Check sheet for the modelled part. Datum: model origin and axes. Units: mm. Face numbers are marked on the shaded views. A direction names the side the tool comes from. Round coordinates to 2 decimals unless told otherwise and drop trailing zeros. One line per question, with ' | ' between items.
Autodesk Inventor part; units mm, degrees
ref_plane "YZ Plane" through (0, 0, 0) normal (1, 0, 0) x (0, 1, 0)
ref_plane "XZ Plane" through (0, 0, 0) normal (0, 1, 0) x (-1, 0, 0)
ref_plane "XY Plane" through (0, 0, 0) normal (0, 0, 1) x (1, 0, 0)
sketch "Skizze1" plane through (0, 0, 0) normal (0, 0, 1) x (1, 0, 0)
  line L0 (-91, 0) -> (91, 0) construction
  circle A0 centre (0, 0) radius 65
  line L1 (-9.5, 25) -> (9.5, 25)
  line L2 (9.5, 25) -> (9.5, 22)
  line L3 (9.5, 22) -> (-9.5, 22)
  line L4 (-9.5, 22) -> (-9.5, 25)
  line L5 (1.5, 22) -> (-1.5, 22)
  line L6 (-1.5, 22) -> (-1.5, 15)
  line L7 (-1.5, 15) -> (1.5, 15)
  line L8 (1.5, 15) -> (1.5, 22)
  circle A1 centre (0, 0) radius 10
  line L9 (0, 91) -> (0, -91) construction
  dimension "d9" = 130
  dimension "d10" = 3
  dimension "d14" = 19
  dimension "d23" = 7
  dimension "d62" = 20
  dimension "d149" = 25
extrude "Extrusion3" add sketch "Skizze1" against normal blind 7 contours L1 L2 L3 L4 | L3 L8 L7 L6
chamfer "Fase2" distance 3 distance2 7 1 edges at (-9.5, 23.5, -7) measured on face at (-0.5, 24, -7)
chamfer "Fase3" distance 3 distance2 7 1 edges at (9.5, 23.5, -7) measured on face at (1.5, 24, -7)
fillet "Rundung1" radius 4 2 edges at (-6.5001, 23.5, -7) (6.5001, 23.5, -7)
sketch "Skizze2" plane through (-9.5, 25, 0) normal (0, 1, 0) x (1, 0, 0)
  circle A0 centre (6, 4) radius 0.9
  circle A1 centre (13, 4) radius 0.9
  line L0 (43, 0) -> (-27, 0) construction
  line L1 (-1.6221, 4) -> (19.0112, 4) construction
  line L2 (3, 7) -> (16, 7) construction
  line L3 (0, 0) -> (0, 3)
  line L4 (9.5, 8.4) -> (9.5, -1.4) construction
  point P0 (9.5, 0)
  point P1 (4, 7)
  point P2 (11, 7)
  dimension "d16" = 1.8
  dimension "d20" = 3
  dimension "d150" = 7
extrude "Extrusion4" cut sketch "Skizze2" against normal up to next
chamfer "Fase1" distance 7 distance2 7 1 edges at (0, 15, -7) measured on face at (0.5, 24, -7)
pattern_circular "Runde Anordnung1" count 3 over 360 about axis through (0, 0, -10) along (0, 0, 1) of "Extrusion4", "Extrusion3", "Fase2", "Fase3", "Rundung1", "Fase1"
extrude "Extrusion11" add sketch "Skizze1" along normal blind 2 contours A0 | L1 L2 L3 L4 | L3 L8 L7 L6
fillet "Rundung5" radius 1 4 edges at (-65, 0, 2) (-10, 0, 2) (-10, 0, 0) (-65, 0, 0)
properties part number "Stewart-Plate-Head"
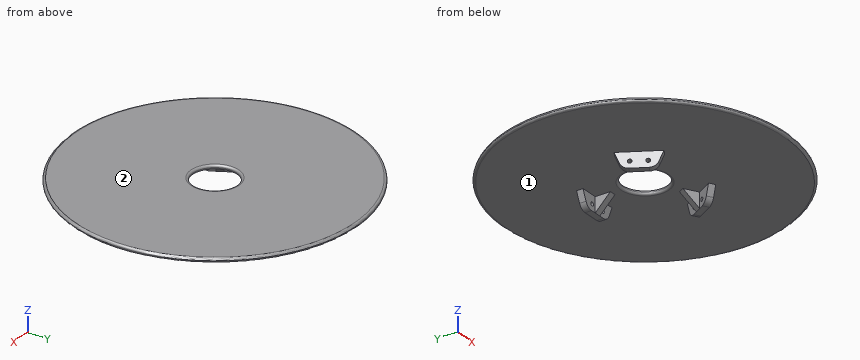
(1) Go/stop test with flat-tipped pins: pin 1 (1.6 mm diameter, centred on x = -3.5, z = -4, fed in from +Y); pin 2 (2 mm diameter, centred on x = 1, z = -2.5, fed in from -Y); pin 3 (3.5 mm diameter, centred on x = 3.5, z = -5, fed in from +Y); pin 4 (2 mm diameter, centred on y = 20, z = -3.5, fed in from +X). Record where each tip stops, or that it passes through.
Answer:
pin 1: passes through | pin 2: stops at y = 16.5 | pin 3: stops at y = 25 | pin 4: stops at x = 1.5
(2) Scan lines: probe 1 along X at (y, z) = (23.7, -4); probe 2 along Z at (x, y) = (3.5, 24.1); probe 3 along Y at (x, z) = (0, 1). Record each from-to range of solid material in increasing order.
Answer:
probe 1: x = -7.79 to -4.4, -2.6 to 2.6, 4.4 to 7.79 | probe 2: z = -7 to -4.9, -3.1 to 2 | probe 3: y = -65 to -10, 10 to 65
(3) Set-up check for the marked faces 1 and 2: record each of +Z, -Z, +X, -X, +Y, -Y from which the full face is reachable in a straight line by a thin tool's end or side.
Answer:
face 1: -Z | face 2: +Z, +X, -X, +Y, -Y
